from build123d import *

# Parameters (mm, degrees)
SKETCH1_R           = 38.5
SKETCH1_R_2         = 28.5
BOSS_EXTRUDE1_DEPTH = 3
SKETCH3_R           = 38.5
BOSS_EXTRUDE2_DEPTH = 5
SKETCH4_W           = 5
SKETCH4_H           = 20
BOSS_EXTRUDE3_DEPTH = 25
SKETCH5_W           = 105
SKETCH5_H           = 20
BOSS_EXTRUDE4_DEPTH = 3
SKETCH6_W           = 2.8
SKETCH6_H           = 20
BOSS_EXTRUDE5_DEPTH = 16
SKETCH7_W           = 8.2
SKETCH7_H           = 20
BOSS_EXTRUDE6_DEPTH = 50
SKETCH8_W           = 11.8
SKETCH8_H           = 23
CUT_EXTRUDE1_DEPTH  = 50
SKETCH9_R           = 2.5
CUT_EXTRUDE2_DEPTH  = 50
SKETCH10_R          = 0.5
CUT_EXTRUDE3_DEPTH  = 1


with BuildPart() as part:
    # Sketch1 → Boss-Extrude1 (new body)
    with BuildSketch(Plane(origin=(0, 0, 0), x_dir=(1, 0, 0), z_dir=(0, 1, 0))):
        Circle(SKETCH1_R)
        Circle(SKETCH1_R_2, mode=Mode.SUBTRACT)
    extrude(amount=BOSS_EXTRUDE1_DEPTH)

    # Sketch3 → Boss-Extrude2 (add)
    with BuildSketch(Plane(origin=(0, 3, 0), x_dir=(1, 0, 0), z_dir=(0, 1, 0))):
        Circle(SKETCH3_R)
    extrude(amount=BOSS_EXTRUDE2_DEPTH)

    # Sketch4 → Boss-Extrude3 (add)
    with BuildSketch(Plane(origin=(0, 8, 0), x_dir=(1, 0, 0), z_dir=(0, 1, 0))):
        with Locations((-32.5, 0)):
            Rectangle(SKETCH4_W, SKETCH4_H)
        with Locations((32.5, 0)):
            Rectangle(SKETCH4_W, SKETCH4_H)
    extrude(amount=BOSS_EXTRUDE3_DEPTH)

    # Sketch5 → Boss-Extrude4 (add)
    with BuildSketch(Plane(origin=(0, 33, 0), x_dir=(1, 0, 0), z_dir=(0, 1, 0))):
        Rectangle(SKETCH5_W, SKETCH5_H)
    extrude(amount=BOSS_EXTRUDE4_DEPTH)

    # Sketch6 → Boss-Extrude5 (add)
    with BuildSketch(Plane(origin=(0, 36, 0), x_dir=(1, 0, 0), z_dir=(0, 1, 0))):
        with Locations((-51.1, 0)):
            Rectangle(SKETCH6_W, SKETCH6_H)
        with Locations((51.1, 0)):
            Rectangle(SKETCH6_W, SKETCH6_H)
    extrude(amount=BOSS_EXTRUDE5_DEPTH)

    # Sketch7 → Boss-Extrude6 (add)
    with BuildSketch(Plane(origin=(0, 36, 0), x_dir=(1, 0, 0), z_dir=(0, 1, 0))):
        with Locations((-45.6, 0)):
            Rectangle(SKETCH7_W, SKETCH7_H)
        with Locations((45.6, 0)):
            Rectangle(SKETCH7_W, SKETCH7_H)
    extrude(amount=BOSS_EXTRUDE6_DEPTH)

    # Sketch8 → Cut-Extrude1 (cut)
    with BuildSketch(Plane.ZY.offset(49.7)):
        with Locations((0, 68.5)):
            Rectangle(SKETCH8_W, SKETCH8_H)
    extrude(amount=-CUT_EXTRUDE1_DEPTH, mode=Mode.SUBTRACT)

    # Sketch9 → Cut-Extrude2 (cut)
    with BuildSketch(Plane.ZY.offset(-41.5)):
        with Locations((0, 74.47)):
            Circle(SKETCH9_R)
    extrude(amount=-CUT_EXTRUDE2_DEPTH, mode=Mode.SUBTRACT)

    # Sketch10 → Cut-Extrude3 (cut)
    with BuildSketch(Plane.XZ.offset(-3)):
        with BuildLine():
            Line((2, 7.5), (2, 2.88735269))
            Line((2, 2.88735269), (17.117647059, 1.996536794))
            ThreePointArc((17.117647059, 1.996536794), (19, 0), (17.117647059, -1.996536794))
            Line((17.117647059, -1.996536794), (2, -2.88735269))
            Line((2, -2.88735269), (2, -7.5))
            ThreePointArc((2, -7.5), (0, -9.5), (-2, -7.5))
            Line((-2, -7.5), (-2, -2.88735269))
            Line((-2, -2.88735269), (-17.117647059, -1.996536794))
            ThreePointArc((-17.117647059, -1.996536794), (-19, 0), (-17.117647059, 1.996536794))
            Line((-17.117647059, 1.996536794), (-2, 2.88735269))
            Line((-2, 2.88735269), (-2, 7.5))
            ThreePointArc((-2, 7.5), (0, 9.5), (2, 7.5))
        make_face()
        with Locations((-17, 0)):
            Circle(SKETCH10_R, mode=Mode.SUBTRACT)
        with Locations((17, 0)):
            Circle(SKETCH10_R, mode=Mode.SUBTRACT)
        with Locations((0, 7.5)):
            Circle(SKETCH10_R, mode=Mode.SUBTRACT)
        with Locations((0, -7.5)):
            Circle(SKETCH10_R, mode=Mode.SUBTRACT)
    extrude(amount=-CUT_EXTRUDE3_DEPTH, mode=Mode.SUBTRACT)


solid = part.part
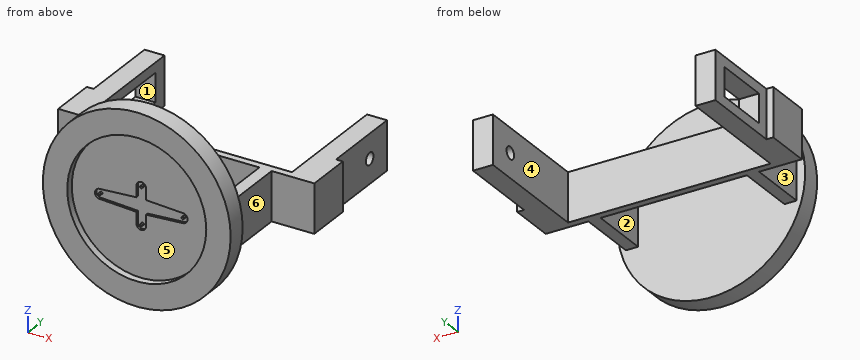
Can you work these out from the model? Positions are in its coordinate system, mm. Face numbers are marked on the shaded views. A direction names the side the tool comes from. Coordinates: 2 decimals unless noted, no trailing zeros. Loops run counter-clockwise (first coordinate to the right, second up) from the corner with the lowest first, then second, coordinate; pieces in that order, holes last. Notation, with made-up numbers: (12, 57) - (60, 57) arc R18 cw to (60, 81) - close; hole circle Ø9 at (79, 32). An arc over 180 degrees is marked (long way). Answer as a JSON object with one key per item and string values. Group by question number.
Item 1: For pin 1 (2 mm diameter, centred on x = -50.5, z = 1.5, fed in from +Y); pin 2 (1.1 mm diameter, centred on y = 3.5, z = -5, fed in from -X); pin 3 (0.5 mm diameter, centred on x = 0, z = 7.5, fed in from -Y); pin 4 (1.5 mm diameter, centred on y = 66.5, z = -6.5, fed in from -X), each with a flat end and sliding along its axis, tell me the tip position at first contact or that it passes through.
Item 2: If we section it at C-C (y = 60): List the corners of the cut face in (x, z) for me.
Item 3: On a 3-axis mill with a long thin cutter (end or side, diameter ignored), from which of +Z, -Z, +X, -X, +Y, -Y can I reach the whole of each face in a straight line? I mean the marked faces 1, 2 and 3. Say none if no direction works.
Item 4: If we mould it in two halves opening along Y, with no side actions, what happens to the marked faces 4, 5 and 6? For each: released by +Y, released by -Y, zero draft, split by the parting line, or undercut.
Item 5: If we section it at B-B (y = 74.47): List the corners of the cut face in (x, z) for me.
Item 6: If I drill on L1, parallel to Y at x = -20.5, z = -2; L2, parallel to X at y = 29, z = 8.5; L3, parallel to Z at x = 0, y = 2, over which ranges is the centre line in solid material (lowest first)? Write a range as from..to.
Item 7: If we section it at A-A (y = 22): List the corners of the cut face in (x, z) for me.
Item 8: If we section it at D-D (z = 13.5): List the corners of the cut face in (x, y) for me.
Returned:
{
 "1": {"pin 1": "stops at y = 86", "pin 2": "stops at x = -38.24", "pin 3": "stops at y = 3", "pin 4": "stops at x = -49.7"},
 "2": {"outline": "(-49.7, -10) - (-41.5, -10) - (-41.5, -5.9) - (-49.7, -5.9) - close; (-49.7, 5.9) - (-41.5, 5.9) - (-41.5, 10) - (-49.7, 10) - close; (41.5, -10) - (49.7, -10) - (49.7, 10) - (41.5, 10) - close"},
 "3": {"face 1": "-X", "face 2": "+Z, -Z", "face 3": "+Z, -Z, -X"},
 "4": {"face 4": "zero draft", "face 5": "released by -Y", "face 6": "undercut"},
 "5": {"outline": "(-49.7, -10) - (-41.5, -10) - (-41.5, -5.9) - (-49.7, -5.9) - close; (-49.7, 5.9) - (-41.5, 5.9) - (-41.5, 10) - (-49.7, 10) - close; (41.5, -10) - (49.7, -10) - (49.7, -2.5) - (41.5, -2.5) - close; (41.5, 2.5) - (49.7, 2.5) - (49.7, 10) - (41.5, 10) - close"},
 "6": {"L1": "y = 3..8, 33..36", "L2": "x = -35..-30, 30..35", "L3": "z = -38.5..-28.5, 28.5..38.5"},
 "7": {"outline": "(-35, -10) - (-30, -10) - (-30, 10) - (-35, 10) - close; (30, -10) - (35, -10) - (35, 10) - (30, 10) - close"},
 "8": {"outline": "(-36.06, 0) - (-25.1, 0) - (-25.1, 3) - (25.1, 3) - (25.1, 0) - (36.06, 0) - (36.06, 8) - (-36.06, 8) - close"}
}
